from build123d import *

# Parameters (mm, degrees)
SKETCH1_R           = 10
BOSS_EXTRUDE1_DEPTH = 4
SKETCH2_R           = 2.45
CUT_EXTRUDE1_DEPTH  = 2.5
SKETCH3_W           = 20
SKETCH3_H           = 15
SKETCH3_R           = 3
BOSS_EXTRUDE2_DEPTH = 10
SKETCH4_R           = 1.4
CUT_EXTRUDE2_DEPTH  = 8


with BuildPart() as part:
    # Sketch1 → Boss-Extrude1 (new body)
    with BuildSketch(Plane(origin=(0, 0, 0), x_dir=(1, 0, 0), z_dir=(0, 1, 0))):
        with Locations(Location((0, 0, 0), (0, 0, 270))):
            Circle(SKETCH1_R)
    extrude(amount=BOSS_EXTRUDE1_DEPTH)

    # Sketch2 → Cut-Extrude1 (cut)
    with BuildSketch(Plane.XZ):
        with Locations(Location((0, 0, 0), (0, 0, 270))):
            Circle(SKETCH2_R)
    extrude(amount=-CUT_EXTRUDE1_DEPTH, mode=Mode.SUBTRACT)

    # Sketch3 → Boss-Extrude2 (add, symmetric)
    with BuildSketch(Plane(origin=(0, 0, 0), x_dir=(0, 0, -1), z_dir=(1, 0, 0))):
        with Locations((0, 11.5)):
            Rectangle(SKETCH3_W, SKETCH3_H)
        with Locations((0, 11.5)):
            Circle(SKETCH3_R, mode=Mode.SUBTRACT)
    extrude(amount=BOSS_EXTRUDE2_DEPTH, both=True)

    # Sketch4 → Cut-Extrude2 (cut)
    with BuildSketch(Plane(origin=(0, 19, 0), x_dir=(1, 0, 0), z_dir=(0, 1, 0))):
        with Locations(Location((0, 0, 0), (0, 0, 270))):
            Circle(SKETCH4_R)
    extrude(amount=-CUT_EXTRUDE2_DEPTH, mode=Mode.SUBTRACT)


solid = part.part
Read the model definition and answer for the solid it produces. Units are mm, in the model's axes. A direction names the side the tool comes from. Coordinates: 2 decimals unless noted, no trailing zeros. Order: outer loops, then holes, each group sorted by start corner. A loop starts at its lowest first (then second) coordinate and runs counter-clockwise, first axis right, second up. Notation, with made-up numbers: (-15, -34) -> (38, -34) arc R29 ccw to (38, 5) -> close; hole circle Ø5 at (-32.5, -20). An arc over 180 degrees is marked (long way). Answer as a JSON object with one key per item and string values.
1) A cutting plane is placed at D-D, the plane y = 15.5. Determine the outline of the cut face in (x, z), plus the area to 3 significant figures.
Model answer:
{"outline": "(-10, -10) -> (10, -10) -> (10, 10) -> (-10, 10) -> close; hole circle Ø2.8 at (0, 0)", "area": "394 mm²"}
2) Consider line 1 along X through (y, z) = (1.25, 0); line 2 along X through (y, z) = (16.4, 0). Determine where each line is inside the solid, lowest interval first. Write a range as from..to.
Model answer:
{"line 1": "x = -10..-2.45, 2.45..10", "line 2": "x = -10..-1.4, 1.4..10"}
3) A cutting plane is placed at B-B, the plane z = -0.5. State how many separate pieces and enclosed holes the cut face has, plus the area to 3 significant figures.
Model answer:
{"separate pieces": "3", "enclosed holes": "0", "area": "238 mm²"}
4) A cutting plane is placed at C-C, the plane x = 5.5. Determine the outline of the cut face in (y, z).
Model answer:
{"outline": "(0, -8.35) -> (4, -8.35) -> (4, -10) -> (19, -10) -> (19, 10) -> (4, 10) -> (4, 8.35) -> (0, 8.35) -> close; hole circle Ø6 at (11.5, 0)"}
5) A tool of negligible diameter and unlimited length cuts with its end or side. For faces 1 (the face through (-8, 4, 8)), 2 (the face through (-8, 4, -8)), 3 (the face through (0.421, 16.611, 1.335)), 4 (the face through (8, 4, -8)), from which of +Z, -Z, +X, -X, +Y, -Y can it reach the whole face along a straight path? Write none if from no direction.
Model answer:
{"face 1": "+Z, -X, -Y", "face 2": "-Z, -X, -Y", "face 3": "+Y", "face 4": "-Z, +X, -Y"}
6) This flat-tipped pin is pushed along its axis until it touches: pin 1 (4 mm diameter, centred on x = 0, z = 0, fed in from -Y). Where does it stop, or does it pass through?
Model answer:
{"pin 1": "stops at y = 2.5"}
7) A cutting plane is placed at A-A, the plane y = 11.5. Determine the outline of the cut face in (x, z), plus the area to 3 significant figures.
Model answer:
{"outline": "(-10, -10) -> (10, -10) -> (10, -3) -> (-10, -3) -> close; (-10, 3) -> (10, 3) -> (10, 10) -> (-10, 10) -> close", "area": "280 mm²"}
8) The mould has two halves that part along X. Classify faces 5 (the face through (0.736, 1.232, -2.337)), 6 (the face through (10, 15, 0)), 7 (the face through (8, 4, 8)), 8 (the face through (0, 2.5, 0)): released by +X, released by -X, zero draft, split by the parting line, or undercut.
Model answer:
{"face 5": "undercut", "face 6": "released by +X", "face 7": "zero draft", "face 8": "undercut"}
